from build123d import *

# Parameters (mm, degrees)
F1_DEPTH = 2
F3_DEPTH = 1
F4_R     = 0.49999


# Not quite as in the source:
# - a fillet or chamfer is up to 0.001 mm smaller than in the source, because OpenCascade refuses the exact size
# - a feature names something its author has since deleted; it is built from what else it names


with BuildPart() as f1:
    # F0 (on Top) → F1 (new body)
    with BuildSketch(Plane.XY):
        with BuildLine():
            ThreePointArc((23.6934297445, 1.7622585683), (24.2075786729, 10), (23.6934297445, 18.2377414317))
            ThreePointArc((23.6934297445, 18.2377414317), (23.0323232276, 19.4886170119), (21.7089512216, 19.9890548979))
            Line((21.7089512216, 19.9890548979), (1.7932879128, 19.9890548979))
            ThreePointArc((1.7932879128, 19.9890548979), (0.4729381343, 19.491278737), (-0.1901730003, 18.2457313605))
            ThreePointArc((-0.1901730003, 18.2457313605), (-0.7214911689, 10), (-0.1901730003, 1.7542686395))
            ThreePointArc((-0.1901730003, 1.7542686395), (0.4729381343, 0.508721263), (1.7932879128, 0.0109451021))
            Line((1.7932879128, 0.0109451021), (21.7089512216, 0.0109451021))
            ThreePointArc((21.7089512216, 0.0109451021), (23.0323232276, 0.5113829881), (23.6934297445, 1.7622585683))
        make_face()
    extrude(amount=F1_DEPTH)

    # F2 (on face) → F3 (join)
    with BuildSketch(Plane.XY.offset(2)):
        with BuildLine():
            Line((21.7089512216, 19.4890548979), (1.7932879128, 19.4890548979))
            ThreePointArc((1.7932879128, 19.4890548979), (0.8030255789, 19.1157227772), (0.305692228, 18.1815622449))
            ThreePointArc((0.305692228, 18.1815622449), (-0.2214911689, 10), (0.305692228, 1.8184377551))
            ThreePointArc((0.305692228, 1.8184377551), (0.8030255789, 0.8842772228), (1.7932879128, 0.5109451021))
            Line((1.7932879128, 0.5109451021), (21.7089512216, 0.5109451021))
            ThreePointArc((21.7089512216, 0.5109451021), (22.7014802261, 0.8862735166), (23.1973101138, 1.8244302017))
            ThreePointArc((23.1973101138, 1.8244302017), (23.7075786729, 10), (23.1973101138, 18.1755697983))
            ThreePointArc((23.1973101138, 18.1755697983), (22.7014802261, 19.1137264834), (21.7089512216, 19.4890548979))
        make_face()
    extrude(amount=F3_DEPTH)

    # F4 (radius 0.5 in the source; OpenCascade refuses exactly that, so slightly less here)
    f4_edges = [f1.edges().sort_by_distance(p)[0] for p in [
        (11.75112, 0.010945, 2),
        (11.75112, 19.989055, 2),
        (23.032323, 0.511383, 2),
        (0.472938, 0.508721, 2),
        (24.207579, 10, 2),
        (-0.721491, 10, 2),
        (0.472938, 19.491279, 2),
        (23.032323, 19.488617, 2),
        (11.75112, 0.510945, 3),
        (0.803026, 0.884277, 3),
        (-0.221491, 10, 3),
        (11.75112, 19.489055, 3),
        (22.70148, 19.113726, 3),
        (23.707579, 10, 3),
        (0.803026, 19.115723, 3),
        (22.70148, 0.886274, 3),
    ]]
    fillet(f4_edges, radius=F4_R)


solid = f1.part
Geometry: final body of the model. Coordinates: model frame, mm. A direction names the side the tool comes from. Round coordinates to 2 decimals unless told otherwise and drop trailing zeros. Loops run counter-clockwise (first coordinate to the right, second up) from the corner with the lowest first, then second, coordinate; pieces in that order, holes last. Notation, with made-up numbers: M -20,-28 L 26,-28 A18 ccw 26,4 Z; hole C -15,39.25 d7. An arc over 180 degrees is marked long. Put each result on its own line as item: value. Start each with the question number.
(1) Material intervals for line 1 along Y through (x, z) = (6.5, 1.55); line 2 along X through (y, z) = (1.75, 1.45); line 3 along X through (y, z) = (14.25, 1.6), sorted ascending. Write a range as [from, to].
(2) Contact query for flat-ended pins moving along their axis: pin 1 Ø0.6 at (x, z) = (8.5, 2) entering from -Y; pin 2 Ø0.6 at (x, z) = (15, 2.5) entering from +Y; pin 3 Ø1.5 at (x, y) = (15, 3) entering from -Z. Output: stop coordinate, or through.
(3) Set-up query: faces 1 (the face through (22.713, 19.104, 2.247)), 2 (the face through (22.69, 0.876, 2.247)), 3 (the face through (0.792, 0.894, 2.247)), 4 (the face through (23.047, 19.475, 0.74)), 5 (the face through (0.814, 19.126, 2.247)). Return all of +Z, -Z, +X, -X, +Y, -Y with unobstructed straight access to the full face (end or side cutting, diameter ignored); none if empty.
(4) Section query B-B (z = 0.65). Return loops of the section in (x, y), then the cut area to 3 significant figures.
Findings below:
1. line 1: y = [0.01, 19.99]
1. line 2: x = [-0.19, 23.69]
1. line 3: x = [-0.57, 24.06]
2. pin 1: stops at y = 0.05
2. pin 2: stops at y = 19.49
2. pin 3: stops at z = 0
3. face 1: +Z, +X, +Y
3. face 2: +Z, +X, -Y
3. face 3: +Z, -X, -Y
3. face 4: +Z, -Z, +X, +Y
3. face 5: +Z, -X, +Y
4. outline: M -0.19,1.75 A2 ccw 1.79,0.01 L 21.71,0.01 A2 ccw 23.69,1.76 A66.25 ccw 23.69,18.24 A2 ccw 21.71,19.99 L 1.79,19.99 A2 ccw -0.19,18.25 A64.25 ccw Z
4. area: 485 mm2
